Design review of the part shown in the three views and the two pictorial views. Dimensions are in mm from the part's minimum x, y and z. A direction names the side the tool comes from. Round coordinates to 2 decimals unless told otherwise and drop trailing zeros. Order: outer loops, then holes, each group sorted by start corner. A loop starts at its lowest first (then second) coordinate and runs counter-clockwise, first axis right, second up. Notation, with made-up numbers: (16.25, 10) - (41.25, 10) arc R10 ccw to (41.25, 24) - close; hole circle Ø1 at (-28.75, 8). An arc over 180 degrees is marked (long way). One line per question, with ' | ' between items. Start each with the question number.
Item 1: Add section B-B on x = 7.12. State the section outline as (y, z) points, and give its area (3 significant figures).
Item 2: Insertion check: pin 1 Ø5.5 at (x, y) = (12.5, 2) entering from -Z; pin 2 Ø3.5 at (x, z) = (18.5, 5.5) entering from -Y; pin 3 Ø6 at (y, z) = (2, 5.5) entering from -X; pin 4 Ø2.5 at (x, y) = (18.5, 4.5) entering from -Z. Each pin has a flat end and moves straight along its axis. Give the tip position at first contact, or say it passes through.
Item 3: For L1, parallel to X at y = 6.5, z = 19; L2, parallel to X at y = 8.55, z = 2; L3, parallel to Z at x = 2.5, y = 3.5 (3 decimals), list the stretches that pass through material, from the lowest coordinate up. Write a range as [from, to].
Item 4: Add section D-D on z = 10. State the section outline as (x, y) points, and give its area (3 significant figures).
Item 5: Add section C-C on y = 1.5. State the section outline as (x, z) points (3 decimals), and give its area (3 significant figures).
Item 6: Draft analysis for pull direction Z (two halves, no side actions). For the marked faces 3, 4, 5 and 6, state which applies: +Z half, -Z half, draft (parallel to the pull), parting line (faces both ways), or undercut.
Item 7: Add section A-A on z = 18. State the section outline as (x, y) points.
Item 8: Tool access review of the marked faces 1 and 2: name each direction out of +Z, -Z, +X, -X, +Y, -Y from which nothing blocks a thin tool from reaching the whole face with its end or side.
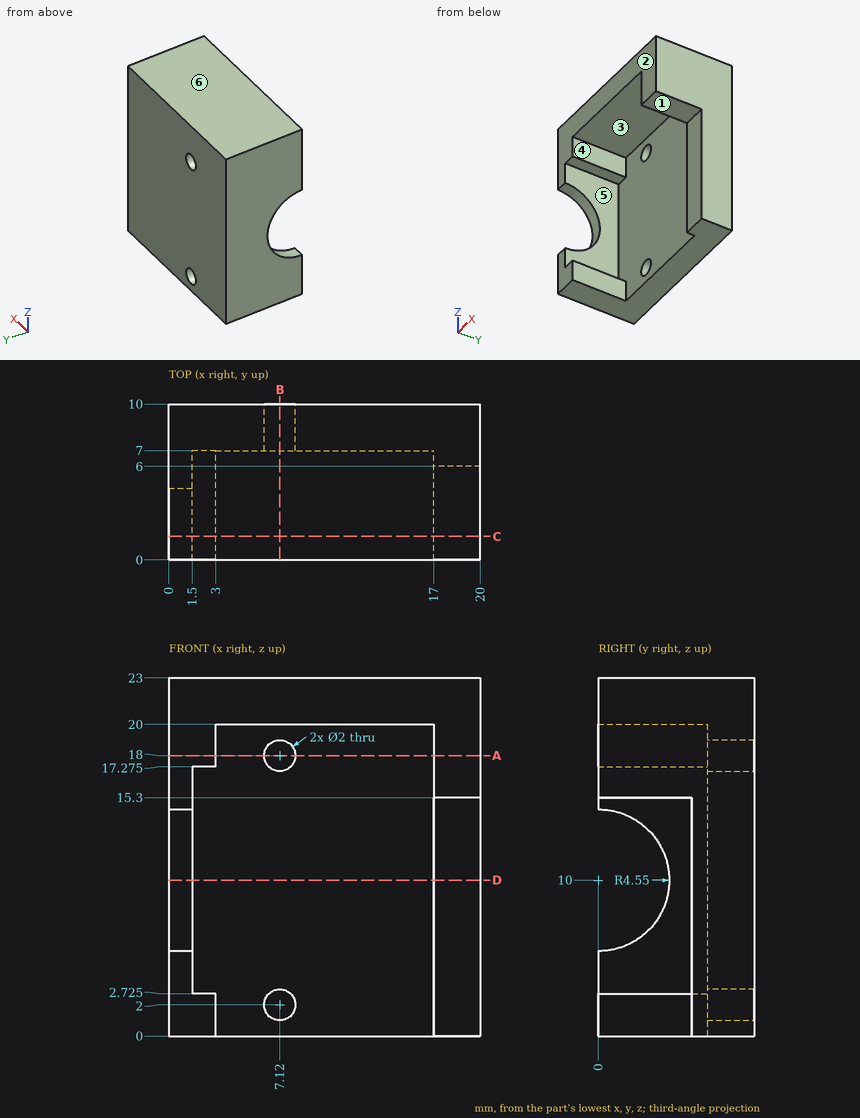
Determined:
1) outline: (0, 20) - (7, 20) - (7, 19) - (10, 19) - (10, 23) - (0, 23) - close; (7, 0) - (10, 0) - (10, 1) - (7, 1) - close; (7, 3) - (10, 3) - (10, 17) - (7, 17) - close | area: 78.0 mm2
2) pin 1: z = 20 | pin 2: y = 6 | pin 3: x = 0 | pin 4: z = 15.3
3) L1: [0, 3], [17, 20] | L2: [0, 6.12], [8.12, 20] | L3: [0, 2.725], [17.275, 23]
4) outline: (0, 4.55) - (1.5, 4.55) - (1.5, 7) - (17, 7) - (17, 6) - (20, 6) - (20, 10) - (0, 10) - close | area: 66.7 mm2
5) outline: (0, 0) - (3, 0) - (3, 2.725) - (1.5, 2.725) - (1.5, 5.704) - (0, 5.704) - close; (0, 14.296) - (1.5, 14.296) - (1.5, 17.275) - (3, 17.275) - (3, 20) - (17, 20) - (17, 15.3) - (20, 15.3) - (20, 23) - (0, 23) - close | area: 99.4 mm2
6) face 3: -Z half | face 4: draft | face 5: undercut | face 6: +Z half
7) outline: (0, 0) - (3, 0) - (3, 7) - (6.12, 7) - (6.12, 10) - (0, 10) - close; (8.12, 7) - (17, 7) - (17, 0) - (20, 0) - (20, 10) - (8.12, 10) - close
8) face 1: -Z, +X, -Y | face 2: +Z, -Z, +X, -X, -Y
